Autodesk Inventor part; units mm, degrees
ref_plane "YZ Plane" through (0, 0, 0) normal (1, 0, 0) x (0, 1, 0)
ref_plane "XZ Plane" through (0, 0, 0) normal (0, 1, 0) x (-1, 0, 0)
ref_plane "XY Plane" through (0, 0, 0) normal (0, 0, 1) x (1, 0, 0)
sketch "Sketch1" plane through (0, 0, 0) normal (0, 1, 0) x (-1, 0, 0)
  line L0 (52.3087, -21.6726) -> (-32.6913, -21.6726)
  line L1 (-32.6913, -21.6726) -> (-32.6913, 48.3274)
  line L2 (-32.6913, 48.3274) -> (52.3087, 48.3274)
  line L3 (52.3087, 48.3274) -> (52.3087, -21.6726)
  dimension "d4" = 70
  dimension "d5" = 85
extrude "Extrusion1" add sketch "Sketch1" along normal blind 33
sketch "Sketch2" plane through (0, 33, 0) normal (0, 1, 0) x (1, 0, 0)
  line L0 (32.6913, 21.6726) -> (-52.3087, 21.6726)
  line L1 (-52.3087, 21.6726) -> (-52.3087, -48.3274)
  line L2 (-52.3087, -48.3274) -> (32.6913, -48.3274)
  line L3 (32.6913, -48.3274) -> (32.6913, 21.6726)
  line L4 (-52.3087, 21.6726) -> (32.6913, 21.6726)
  line L5 (32.6913, 21.6726) -> (32.6913, -43.3274)
  line L6 (32.6913, -43.3274) -> (-52.3087, -43.3274)
  line L7 (-52.3087, -43.3274) -> (-52.3087, 21.6726)
  point P0 (0, 0)
  dimension "d8" = 0
  dimension "d9" = 0
  dimension "d10" = 5
extrude "Extrusion2" cut sketch "Sketch2" against normal blind 25 contours L3 L6 L1 L0
sketch "Sketch3" plane through (0, 8, 0) normal (0, 1, 0) x (1, 0, 0)
  line L0 (32.6913, -43.3274) -> (-52.3087, -43.3274)
  line L1 (-35.8087, 6.6726) -> (16.1913, 6.6726)
  line L2 (16.1913, 6.6726) -> (16.1913, -19.3274)
  line L3 (16.1913, -19.3274) -> (-35.8087, -19.3274)
  line L4 (-35.8087, -19.3274) -> (-35.8087, 6.6726)
  line L5 (-52.3087, 21.6726) -> (32.6913, 21.6726)
  line L6 (-52.3087, -48.3274) -> (-52.3087, 21.6726)
  line L7 (-9.8087, -43.3274) -> (-9.8087, 21.6726) construction
  circle A0 centre (-39.3087, -23.3274) radius 1.75
  circle A1 centre (-39.3087, 10.6726) radius 1.75
  circle A2 centre (19.6913, 10.6726) radius 1.75
  circle A3 centre (19.6913, -23.3274) radius 1.75
  line L8 (-52.6639, -6.3274) -> (32.3361, -6.3274) construction
  point P0 (0, 0)
  dimension "d106" = 26
  dimension "d107" = 3.5
  dimension "d110" = 34
  dimension "d111" = 59
  dimension "d144" = 52
  dimension "d145" = 15
extrude "Extrusion3" cut sketch "Sketch3" against normal blind 1.5
sketch "Sketch4" plane through (0, 6.5, 0) normal (0, 1, 0) x (1, 0, 0)
  line L0 (-35.8087, 6.6726) -> (16.1913, 6.6726)
  line L1 (-35.8087, -19.3274) -> (-35.8087, 6.6726)
  line L2 (16.1913, -19.3274) -> (-35.8087, -19.3274)
  line L3 (16.1913, 6.6726) -> (16.1913, -19.3274)
  line L4 (-33.8087, 4.6726) -> (12.1913, 4.6726)
  line L5 (12.1913, 4.6726) -> (12.1913, -17.3274)
  line L6 (12.1913, -17.3274) -> (-33.8087, -17.3274)
  line L7 (-33.8087, -17.3274) -> (-33.8087, 4.6726)
  point P0 (0, 0)
  dimension "d20" = 2
  dimension "d21" = 2
  dimension "d22" = 2
  dimension "d23" = 4
extrude "Extrusion4" cut sketch "Sketch4" against normal blind 1 contours L4 L5 L6 L7
sketch "Sketch10" plane through (32.6913, 8, 43.3274) normal (0, 0, -1) x (-1, 0, 0)
  line L0 (85, 25) -> (85, 0)
  line L1 (0, 25) -> (85, 25)
  circle A0 centre (18, 9.75) radius 3.5
  circle A1 centre (67, 9.75) radius 3.5
  point P0 (32.6913, -8)
  dimension "d53" = 15.25
  dimension "d55" = 15.25
  dimension "d58" = 7
  dimension "d59" = 7
  dimension "d70" = 49
  dimension "d71" = 18
extrude "Extrusion9" cut sketch "Sketch10" against normal blind 5
sketch "Sketch16" plane through (16.1913, 8, -6.6726) normal (-1, 0, 0) x (0, 0, 1)
  line L0 (0, 0) -> (26, 0)
  line L1 (0, 0) -> (0, -1.5)
  line L2 (0, -1.5) -> (26, -1.5)
  line L3 (26, 0) -> (26, -1.5)
  point P0 (6.6726, -8)
sketch "Sketch17" plane through (0, 5.5, 0) normal (0, 1, 0) x (1, 0, 0)
  line L0 (-33.8087, 4.6726) -> (12.1913, 4.6726)
  line L1 (-33.8087, -17.3274) -> (-33.8087, 4.6726)
  line L2 (12.1913, -17.3274) -> (-33.8087, -17.3274)
  line L3 (12.1913, 4.6726) -> (12.1913, -17.3274)
  line L4 (-33.8087, 4.6726) -> (12.1913, 4.6726)
  line L5 (12.1913, 4.6726) -> (12.1913, -17.3274)
  line L6 (12.1913, -17.3274) -> (-33.8087, -17.3274)
  line L7 (-33.8087, -17.3274) -> (-33.8087, 4.6726)
  point P0 (0, 0)
  dimension "d93" = 0
  dimension "d94" = 0
  dimension "d95" = 0
  dimension "d96" = 0
extrude "Extrusion14" cut sketch "Sketch17" along normal through all both and the other way through all
sketch "Sketch20" plane through (32.6913, 0, 48.3274) normal (1, 0, 0) x (0, 0, -1)
  line L0 (21.875, 5.625) -> (28.125, 5.625)
  line L1 (28.125, 5.625) -> (28.125, 2.375)
  line L2 (28.125, 2.375) -> (21.875, 2.375)
  line L3 (21.875, 2.375) -> (21.875, 5.625)
  line L4 (55.875, 5.625) -> (62.125, 5.625)
  line L5 (62.125, 5.625) -> (62.125, 2.375)
  line L6 (62.125, 2.375) -> (55.875, 2.375)
  line L7 (55.875, 2.375) -> (55.875, 5.625)
  line L8 (25, 6.5) -> (25, 2.375) construction
  line L9 (59, 6.5) -> (59, 2.375) construction
  line L10 (23.25, 6.5) -> (26.75, 6.5) construction
  line L11 (57.25, 6.5) -> (60.75, 6.5) construction
  line L12 (70, 0) -> (70, 8) construction
  line L13 (70, 4) -> (0, 4) construction
  line L14 (0, 0) -> (0, 33) construction
  point P0 (48.3274, 0)
  dimension "d113" = 3.25
  dimension "d125" = 6.25
extrude "Extrusion16" cut sketch "Sketch20" against normal blind 16
sketch "Sketch21" plane through (-52.3087, 0, -21.6726) normal (-1, 0, 0) x (0, 0, 1)
  line L0 (7.875, 5.625) -> (14.125, 5.625)
  line L1 (14.125, 5.625) -> (14.125, 2.375)
  line L2 (14.125, 2.375) -> (7.875, 2.375)
  line L3 (7.875, 2.375) -> (7.875, 5.625)
  line L4 (41.875, 5.625) -> (48.125, 5.625)
  line L5 (48.125, 5.625) -> (48.125, 2.375)
  line L6 (48.125, 2.375) -> (41.875, 2.375)
  line L7 (41.875, 2.375) -> (41.875, 5.625)
  line L8 (7.875, 2.375) -> (14.125, 2.375)
  line L9 (41.875, 2.375) -> (48.125, 2.375)
  line L10 (48.125, 5.625) -> (41.875, 5.625)
  line L11 (41.875, 5.625) -> (41.875, 2.375)
  line L12 (48.125, 2.375) -> (48.125, 5.625)
  line L13 (14.125, 2.375) -> (14.125, 5.625)
  line L14 (7.875, 5.625) -> (7.875, 2.375)
  line L15 (14.125, 5.625) -> (7.875, 5.625)
extrude "Extrusion17" cut sketch "Sketch21" against normal blind 16
sketch "Sketch22" plane through (0, 8, 0) normal (0, 1, 0) x (1, 0, 0)
  circle A0 centre (-39.3087, -23.3274) radius 1.75
  circle A1 centre (19.6913, 10.6726) radius 1.75
  circle A2 centre (-39.3087, 10.6726) radius 1.75
  circle A3 centre (19.6913, -23.3274) radius 1.75
  circle A4 centre (19.6913, 10.6726) radius 1.75
  circle A5 centre (19.6913, -23.3274) radius 1.75
  circle A6 centre (-39.3087, 10.6726) radius 1.75
  circle A7 centre (-39.3087, -23.3274) radius 1.75
  point P0 (0, 0)
extrude "Extrusion18" cut sketch "Sketch22" against normal through all
properties part number "SampleBase"
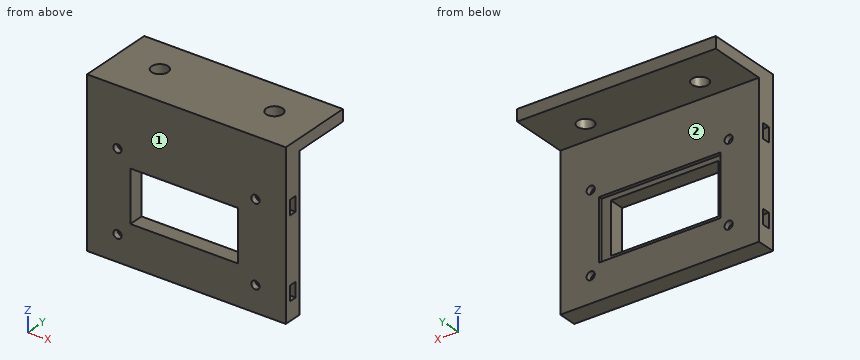
Design review of the part built by this model. Coordinates are the model's own, in mm. Face numbers are marked on the shaded views. A direction names the side the tool comes from. Give positions to 0.01 mm unless a question says otherwise; leave off trailing zeros. Order: outer loops, then holes, each group sorted by start corner. A loop starts at its lowest first (then second) coordinate and runs counter-clockwise, first axis right, second up. Notation, with made-up numbers: (41, -40) -> (70, -40) arc R25 ccw to (70, -6) -> close; hole circle Ø7 at (53, 11). An arc over 180 degrees is marked (long way). Write item = value, one per line. Start each with the question number.
(1) We need section C-C on y = 4.5. Write out the cut boundary in (x, z), plus the area to 3 significant figures.
(2) To check wall thickness, follow line 1 along Y through (x, z) = (-36.5, 24.5) (3 decimals); line 2 along Z through (x, y) = (1, 6); line 3 along X through (y, z) = (17, 46). State the ranges of each line that lie inside material, in increasing order.
(3) We need section B-B on x = -24. Write out the cut boundary in (y, z).
(4) We need section D-D on y = 17.75. Write out the cut boundary in (x, z), plus the area to 3 significant figures.
(5) We need section A-A on z = 6.5. Write out the cut boundary in (x, y).
(6) For pin 1 (4 mm diameter, centred on x = 1, z = 13.5, fed in from -Y); pin 2 (1.6 mm diameter, centred on y = 4.5, z = 24, fed in from -X); pin 3 (4 mm diameter, centred on x = -9.5, z = 25, fed in from +Y); pin 4 (8 mm diameter, centred on x = -26, y = 16, fed in from -Z), all flat-tipped, find the tip position at first contact; note any pin that passes through.
(7) For the marked faces 1 and 2, list the 3-axis set-ups (+Z, -Z, +X, -X, +Y, -Y) from which the entire face can be reached by the end or side of a thin tool; tool diameter is ignored.
Numbers:
q1.outline = (-52.31, -21.67) -> (32.69, -21.67) -> (32.69, -13.8) -> (16.69, -13.8) -> (16.69, -7.55) -> (32.69, -7.55) -> (32.69, 20.2) -> (16.69, 20.2) -> (16.69, 26.45) -> (32.69, 26.45) -> (32.69, 48.33) -> (-52.31, 48.33) -> (-52.31, 26.45) -> (-36.31, 26.45) -> (-36.31, 20.2) -> (-52.31, 20.2) -> (-52.31, -7.55) -> (-36.31, -7.55) -> (-36.31, -13.8) -> (-52.31, -13.8) -> close; hole (-33.81, -4.67) -> (12.19, -4.67) -> (12.19, 17.33) -> (-33.81, 17.33) -> close
q1.area = 4,540 mm^2
q2.line_1 = 0 to 2.375, 5.625 to 8
q2.line_2 = -21.67 to -4.67, 17.33 to 48.33
q2.line_3 = -52.31 to -37.73, -30.89 to 11.27, 18.11 to 32.69
q3.outline = (0, -21.67) -> (8, -21.67) -> (8, -6.67) -> (6.5, -6.67) -> (6.5, -4.67) -> (0, -4.67) -> close; (0, 17.33) -> (6.5, 17.33) -> (6.5, 19.33) -> (8, 19.33) -> (8, 43.33) -> (33, 43.33) -> (33, 48.33) -> (0, 48.33) -> close
q4.outline = (-52.31, 43.33) -> (-37.81, 43.33) -> (-37.81, 48.33) -> (-52.31, 48.33) -> close; (-30.81, 43.33) -> (11.19, 43.33) -> (11.19, 48.33) -> (-30.81, 48.33) -> close; (18.19, 43.33) -> (32.69, 43.33) -> (32.69, 48.33) -> (18.19, 48.33) -> close
q4.area = 355 mm^2
q5.outline = (-52.31, 0) -> (-33.81, 0) -> (-33.81, 6.5) -> (-35.81, 6.5) -> (-35.81, 8) -> (-52.31, 8) -> close; (12.19, 0) -> (32.69, 0) -> (32.69, 8) -> (16.19, 8) -> (16.19, 6.5) -> (12.19, 6.5) -> close
q6.pin_1 = through
q6.pin_2 = -36.31
q6.pin_3 = 8
q6.pin_4 = 43.33
q7.face_1 = +Z, -Z, +X, -X, -Y
q7.face_2 = -Z, +X, -X, +Y
